```python
from build123d import *

# Parameters (mm, degrees)
SKETCH_1_W          = 63.8
SKETCH_1_H          = 7.8
EXTRUDE_1_DEPTH     = 3.2
SKETCH_2_R          = 2.4
EXTRUDE_2_DEPTH     = 1.7
SKETCH_3_R          = 2.5
CUT_EXTRUDE_1_DEPTH = 1.8


with BuildPart() as part:
    # Эскиз1 → Бобышка-Вытянуть1 (new body)
    with BuildSketch(Plane(origin=(0, 0, 0), x_dir=(1, 0, 0), z_dir=(0, 1, 0))):
        Rectangle(SKETCH_1_W, SKETCH_1_H)
    extrude(amount=EXTRUDE_1_DEPTH)

    # Эскиз2 → Бобышка-Вытянуть2 (add)
    with BuildSketch(Plane(origin=(0, 3.2, 0), x_dir=(1, 0, 0), z_dir=(0, 1, 0))):
        with Locations(Location((-28, 0, 0), (0, 0, 270))):
            Circle(SKETCH_2_R)
        with Locations(Location((-20.126, 0, 0), (0, 0, 270))):
            Circle(SKETCH_2_R)
        with Locations(Location((-12.252, 0, 0), (0, 0, 270))):
            Circle(SKETCH_2_R)
        with Locations(Location((-4.378, 0, 0), (0, 0, 270))):
            Circle(SKETCH_2_R)
        with Locations(Location((3.496, 0, 0), (0, 0, 270))):
            Circle(SKETCH_2_R)
        with Locations(Location((11.37, 0, 0), (0, 0, 270))):
            Circle(SKETCH_2_R)
        with Locations(Location((19.244, 0, 0), (0, 0, 270))):
            Circle(SKETCH_2_R)
        with Locations(Location((27.118, 0, 0), (0, 0, 270))):
            Circle(SKETCH_2_R)
    extrude(amount=EXTRUDE_2_DEPTH)

    # Эскиз3 → Вырез-Вытянуть1 (cut)
    with BuildSketch(Plane.XZ):
        with Locations(Location((-28, 0, 0), (0, 0, 270))):
            Circle(SKETCH_3_R)
        with Locations(Location((-20.126, 0, 0), (0, 0, 270))):
            Circle(SKETCH_3_R)
        with Locations(Location((-12.252, 0, 0), (0, 0, 270))):
            Circle(SKETCH_3_R)
        with Locations(Location((-4.378, 0, 0), (0, 0, 270))):
            Circle(SKETCH_3_R)
        with Locations(Location((3.496, 0, 0), (0, 0, 270))):
            Circle(SKETCH_3_R)
        with Locations(Location((11.37, 0, 0), (0, 0, 270))):
            Circle(SKETCH_3_R)
        with Locations(Location((19.244, 0, 0), (0, 0, 270))):
            Circle(SKETCH_3_R)
        with Locations(Location((27.118, 0, 0), (0, 0, 270))):
            Circle(SKETCH_3_R)
    extrude(amount=-CUT_EXTRUDE_1_DEPTH, mode=Mode.SUBTRACT)


solid = part.part
```
Can you work these out from the model? Positions are in its coordinate system, mm. A direction names the side the tool comes from. Give positions to 0.01 mm unless a question says otherwise; leave off trailing zeros. Order: outer loops, then holes, each group sorted by start corner. A loop starts at its lowest first (then second) coordinate and runs counter-clockwise, first axis right, second up. Notation, with made-up numbers: M 34,17.25 L 55,17.25 A20 cw 55,52.25 Z; hole C 1.25,48.5 d9. An arc over 180 degrees is marked long. Write item = value, one per line. Start each with the question number.
Q1. I need wall thicknesses on probe 1 along Y at (x, z) = (-23, 2.25); probe 2 along Z at (x, y) = (11.5, 4.4); probe 3 along Y at (x, z) = (-5, 0). Which ranges of each line are inside material? Lowest first, please. Write a range as [from, to].
Q2. Suppose I cut it at D-D (x = 22.5). Write out the boundary of the cut face in (y, z), plus the area to 3 significant figures.
Q3. Will these pins go through, and if not, where does the flat tip stop? pin 1 Ø1 at (x, y) = (2, 4) entering from +Z; pin 2 Ø1.5 at (x, z) = (-12.5, -1) entering from -Y.
Q4. Suppose I cut it at B-B (z = -3.25). Write out the boundary of the cut face in (x, y), plus the area to 3 significant figures.
Q5. For faces 5 (the cylindrical face through (29.5, 4, -0.3)), 6 (the flat face through (27, 4.9, 0)), 7 (the flat face through (-12, 1.8, 0)), which set-ups out of +Z, -Z, +X, -X, +Y, -Y let a thin tool reach every point of the face, with its end or its side?
Q6. We'd pull the mould along Z, two halves only. Please class faces 1 (the flat face through (4, 1.8, 0)), 2 (the flat face through (0, 3.2, 0)), 3 (the cylindrical face through (21.624, 4.038, -0.312)), 4 (the flat face through (-20, 1.8, 0)): pulls with the +Z half, pulls with the -Z half, needs draft (parallel to the pull), parting line crosses it, or undercut.
Q7. Suppose I cut it at C-C (x = -11.5). Write out the boundary of the cut face in (y, z).
Q8. Suppose I cut it at A-A (x = -28). Write out the boundary of the cut face in (y, z).
Check result:
q1.probe_1 = [0, 3.2]
q1.probe_2 = [-2.4, 2.4]
q1.probe_3 = [1.8, 4.9]
q2.outline = M 0,-3.9 L 3.2,-3.9 L 3.2,3.9 L 0,3.9 Z
q2.area = 25.0 mm2
q3.pin_1 = 2.18
q3.pin_2 = 1.8
q4.outline = M -31.9,0 L 31.9,0 L 31.9,3.2 L -31.9,3.2 Z
q4.area = 204 mm2
q5.face_5 = +Y
q5.face_6 = +Z, -Z, +X, -X, +Y
q5.face_7 = -Y
q6.face_1 = undercut
q6.face_2 = needs draft
q6.face_3 = parting line crosses it
q6.face_4 = undercut
q7.outline = M 0,-3.9 L 3.2,-3.9 L 3.2,-2.28 L 4.9,-2.28 L 4.9,2.28 L 3.2,2.28 L 3.2,3.9 L 0,3.9 L 0,2.38 L 1.8,2.38 L 1.8,-2.38 L 0,-2.38 Z
q8.outline = M 0,-3.9 L 3.2,-3.9 L 3.2,-2.4 L 4.9,-2.4 L 4.9,2.4 L 3.2,2.4 L 3.2,3.9 L 0,3.9 L 0,2.5 L 1.8,2.5 L 1.8,-2.5 L 0,-2.5 Z
